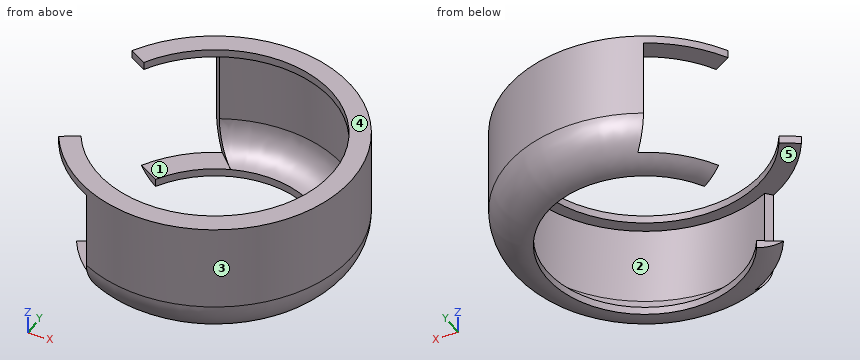
```python
from build123d import *

# Parameters (mm, degrees)
F1_ANGLE = 300
F3_DEPTH = 28


with BuildPart() as f1:
    # F0 (on Front) → F1 (revolve, symmetric)
    with BuildSketch(Plane.XZ) as f1_sk:
        with BuildLine():
            Line((35, -20), (35, 0))
            Line((35, 0), (35, 2))
            Line((35, 2), (30, 2))
            Line((30, 2), (30, 0))
            Line((30, 0), (33, 0))
            Line((33, 0), (33, -20))
            ThreePointArc((33, -20), (30.656854, -25.656854), (25, -28))
            Line((25, -28), (25, -30))
            ThreePointArc((25, -30), (32.071068, -27.071068), (35, -20))
        make_face()
    revolve(axis=Axis((0, 0, -15), (0, 0, -1)), revolution_arc=F1_ANGLE / 2)
    revolve(f1_sk.sketch, axis=Axis((0, 0, -15), (0, 0, 1)), revolution_arc=F1_ANGLE / 2)

    # F2 (on Top) → F3 (cut)
    with BuildSketch(Plane.XY):
        Polygon((-55, -70), (15, 0), (-55, 70), (-55, 0), align=None)
    extrude(amount=-F3_DEPTH, mode=Mode.SUBTRACT)


solid = f1.part
```
Part model, mm, in its own coordinate system. Face numbers are marked on the shaded views. A direction names the side the tool comes from. Round coordinates to 2 decimals unless told otherwise and drop trailing zeros. Loops run counter-clockwise (first coordinate to the right, second up) from the corner with the lowest first, then second, coordinate; pieces in that order, holes last.
Item 1: Drop flat-ended pins along their axis: P1, Ø6, axis at x = 14.5, y = 27.5, coming from the -Z side; P2, Ø5, axis at x = -17.5, z = -18, coming from the +Y side; P3, Ø2, axis at y = 9, z = -15, coming from the -X side. Give the stop position or say it passes through.
Item 2: Mould opens along Y. For the marked faces 3, 4 and 5 say: +Y half, -Y half, draft (parallel to the pull), parting line (faces both ways), or undercut.
Item 3: Cut at D-D, the plane z = -27. Give the cut face in (x, y).
Item 4: Drill centre lines: line 1 (Y direction, x = 0, z = 1); line 2 (Y direction, x = -1.5, z = -18); line 3 (X direction, y = 0, z = -15.75). Where is each one in solid material? Low to high.
Item 5: 3-axis set-ups, long thin cutter, end or side, ignore diameter. For the marked faces 1 and 2: which of +Z, -Z, +X, -X, +Y, -Y reach the whole face in a straight line?
Item 6: Cut at C-C, the plane x = -25. State how many separate pieces and enclosed holes the cut face has, then the cut area to 3 significant figures.
Item 7: Cut at A-A, the plane x = 0. Give the cut face in (y, z).
Item 8: Cut at B-B, the plane y = 0. Give the cut face in (x, z), then the cut area to 3 significant figures.
A:
1. P1: stops at z = -29.51
1. P2: stops at y = 31.62
1. P3: stops at x = 31.45
2. face 3: parting line
2. face 4: draft
2. face 5: undercut
3. outline: (-13.95, -28.95) arc R32.14 ccw (long way) to (-13.95, 28.95) - (-11.49, 26.49) arc R28.87 cw (long way) to (-11.49, -26.49) - close
4. line 1: y = -35 to -30, 30 to 35
4. line 2: y = -34.97 to -32.97, 32.97 to 34.97
4. line 3: x = 33 to 35
5. face 1: -X
5. face 2: none
6. separate pieces: 4
6. enclosed holes: 0
6. area: 37.0 mm2
7. outline: (-35, -20) arc R10 ccw to (-25, -30) - (-25, -28) arc R8 cw to (-33, -20) - (-33, 0) - (-30, 0) - (-30, 2) - (-35, 2) - close; (25, -30) arc R10 ccw to (35, -20) - (35, 2) - (30, 2) - (30, 0) - (33, 0) - (33, -20) arc R8 cw to (25, -28) - close
8. outline: (25, -30) arc R10 ccw to (35, -20) - (35, 2) - (30, 2) - (30, 0) - (33, 0) - (33, -20) arc R8 cw to (25, -28) - close
8. area: 78.3 mm2
